Input: part model. Units: mm. Frame: model coordinates. Face numbers are marked on the shaded views. A direction names the side the tool comes from. Give positions to 0.01 mm unless a question says otherwise; leave off trailing zeros. Loops run counter-clockwise (first coordinate to the right, second up) from the corner with the lowest first, then second, coordinate; pieces in that order, holes last. Notation, with made-up numbers: (55, 26) -> (99, 26) arc R27 ccw to (99, 42) -> close; hole circle Ø8 at (35.25, 37.5). An arc over 180 degrees is marked (long way). Answer in a Markdown table with one row per item. Add a question column.
```python
from build123d import *

# Parameters (mm, degrees)
SKETCH1_R           = 2.25
BOSS_EXTRUDE1_DEPTH = 20
SKETCH2_R           = 2.25
BOSS_EXTRUDE2_DEPTH = 10
SKETCH4_W           = 26.5
SKETCH4_H           = 2.5
CUT_EXTRUDE1_DEPTH  = 39.17921555
CHAMFER2_SIZE       = 4
CHAMFER3_SIZE       = 4
FILLET4_R           = 2
SKETCH7_W           = 10
SKETCH7_H           = 10
BOSS_EXTRUDE5_DEPTH = 20
FILLET6_R           = 2
SKETCH8_W           = 63
SKETCH8_H           = 30
BOSS_EXTRUDE6_DEPTH = 4
CHAMFER4_SIZE       = 2
FILLET7_R           = 2


with BuildPart() as part:
    # Sketch1 → Boss-Extrude1 (new body)
    with BuildSketch(Plane(origin=(0, 0, 0), x_dir=(0, 0, -1), z_dir=(1, 0, 0))):
        Polygon((10.25, -20.3), (13.25, -20.3), (13.25, 29.7), (-13.25, 29.7), (-13.25, -20.3), (-10.25, -20.3), (-10.25, 20.3), (10.25, 20.3), align=None)
        with Locations((5, 24)):
            Circle(SKETCH1_R, mode=Mode.SUBTRACT)
        with Locations((-5, 24)):
            Circle(SKETCH1_R, mode=Mode.SUBTRACT)
    extrude(amount=BOSS_EXTRUDE1_DEPTH)

    # Sketch2 → Boss-Extrude2 (add)
    with BuildSketch(Plane.ZY):
        with Locations((-5, 24)):
            Circle(SKETCH2_R)
        with Locations((5, 24)):
            Circle(SKETCH2_R)
    extrude(amount=-BOSS_EXTRUDE2_DEPTH)

    # Sketch4 → Cut-Extrude1 (cut, through all)
    with BuildSketch(Plane(origin=(20, 0, 0), x_dir=(0, 0, -1), z_dir=(1, 0, 0))):
        with Locations((0, 28.45)):
            Rectangle(SKETCH4_W, SKETCH4_H)
    extrude(amount=-CUT_EXTRUDE1_DEPTH, mode=Mode.SUBTRACT)

    # Chamfer2
    chamfer2_edges = [part.edges().sort_by_distance(p)[0] for p in [
        (10, 27.2, -13.25),
    ]]
    chamfer(chamfer2_edges, length=CHAMFER2_SIZE)

    # Chamfer3
    chamfer3_edges = [part.edges().sort_by_distance(p)[0] for p in [
        (10, 27.2, 13.25),
    ]]
    chamfer(chamfer3_edges, length=CHAMFER3_SIZE)

    # Fillet4
    fillet4_edges = [part.edges().sort_by_distance(p)[0] for p in [
        (10, 27.2, -9.25),
        (10, 27.2, 9.25),
    ]]
    fillet(fillet4_edges, radius=FILLET4_R)

    # Sketch7 → Boss-Extrude5 (add)
    with BuildSketch(Plane(origin=(20, 0, 0), x_dir=(0, 0, -1), z_dir=(1, 0, 0))):
        with Locations((18.25, 6.423218073)):
            Rectangle(SKETCH7_W, SKETCH7_H)
    extrude(amount=-BOSS_EXTRUDE5_DEPTH)

    # Fillet6
    fillet6_edges = [part.edges().sort_by_distance(p)[0] for p in [
        (10, 1.423218073, -13.25),
        (10, 11.423218073, -13.25),
    ]]
    fillet(fillet6_edges, radius=FILLET6_R)

    # Sketch8 → Boss-Extrude6 (add)
    with BuildSketch(Plane(origin=(0, 0, -23.25), x_dir=(-1, 0, 0), z_dir=(0, 0, -1))):
        with Locations((-13.9, 6.423218073)):
            Rectangle(SKETCH8_W, SKETCH8_H)
    extrude(amount=BOSS_EXTRUDE6_DEPTH)

    # Chamfer4
    chamfer4_edges = [part.edges().sort_by_distance(p)[0] for p in [
        (45.4, 6.423218073, -23.25),
        (13.9, -8.576781927, -23.25),
        (-17.6, 6.423218073, -23.25),
        (13.9, 21.423218073, -23.25),
    ]]
    chamfer(chamfer4_edges, length=CHAMFER4_SIZE)

    # Fillet7
    fillet7_edges = [part.edges().sort_by_distance(p)[0] for p in [
        (10, 11.423218073, -23.25),
        (10, 1.423218073, -23.25),
    ]]
    fillet(fillet7_edges, radius=FILLET7_R)


solid = part.part
```
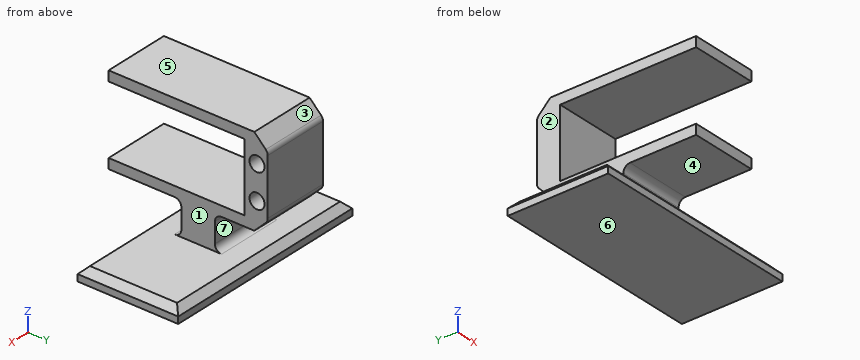
1) Pin query (flat end, axial travel): pin 1 (10 mm diameter, centred on x = 11.5, z = 0, fed in from -Y); pin 2 (1.3 mm diameter, centred on y = 23.5, z = -5, fed in from +X); pin 3 (11 mm diameter, centred on y = 2.5, z = -14, fed in from +X); pin 4 (2 mm diameter, centred on y = 19, z = -4.5, fed in from -X). Return the tip coordinate at first contact, or that it passes through.
2) Section B-B on z = -5. Output: boundary loops of the cut face in (x, y), and give its area (3 significant figures).
3) Pull-direction query (Z, two-part tool) for the marked faces 5, 6 and 7; classes: +Z half, -Z half, draft (parallel to the pull), parting line (faces both ways), or undercut.
4) Section A-A on y = 15. Output: boundary loops of the cut face in (x, z), and give its area (3 significant figures).
5) Section C-C on y = 24. Output: boundary loops of the cut face in (x, z), and give its area (3 significant figures).
6) Material intervals for line 1 along Y through (x, z) = (13.75, 5); line 2 along Z through (x, y) = (8.5, -15); line 3 along Z through (x, y) = (15.5, 24), sorted ascending.
7) Reachability of the marked faces 1, 2, 3 and 4 from +Z, -Z, +X, -X, +Y, -Y: full face, straight path, thin tool, end or side. Return the list, or none.
8) Section D-D on x = -12. Output: boundary loops of the cut face in (y, z), and give its area (3 significant figures).
Working result:
| question | item | result |
|---|---|---|
| 1 | pin 1 | stops at y = 20.3 |
| 1 | pin 2 | stops at x = 10 |
| 1 | pin 3 | stops at x = 20 |
| 1 | pin 4 | passes through |
| 2 | outline | (0, 20.3) -> (20, 20.3) -> (20, 21.75) -> (10, 21.75) -> (10, 26.25) -> (20, 26.25) -> (20, 27.2) -> (0, 27.2) -> close |
| 2 | area | 93.0 mm2 |
| 3 | face 5 | +Z half |
| 3 | face 6 | -Z half |
| 3 | face 7 | undercut |
| 4 | outline | (-17.6, -27.25) -> (45.4, -27.25) -> (45.4, -25.25) -> (43.4, -23.25) -> (-15.6, -23.25) -> (-17.6, -25.25) -> close; (0, -13.25) -> (20, -13.25) -> (20, -10.25) -> (0, -10.25) -> close; (0, 10.25) -> (20, 10.25) -> (20, 13.25) -> (0, 13.25) -> close |
| 4 | area | 368 mm2 |
| 5 | outline | (0, -12.45) -> (20, -12.45) -> (20, -7.25) -> (10, -7.25) -> (10, -2.75) -> (20, -2.75) -> (20, 2.75) -> (10, 2.75) -> (10, 7.25) -> (20, 7.25) -> (20, 12.45) -> (0, 12.45) -> close |
| 5 | area | 408 mm2 |
| 6 | line 1 | y = 20.3 to 21.75, 26.25 to 27.2 |
| 6 | line 2 | z = -13.25 to -10.25, 10.25 to 13.25 |
| 6 | line 3 | z = -12.45 to -7.25, -2.75 to 2.75, 7.25 to 12.45 |
| 7 | face 1 | +Z, +X, +Y, -Y |
| 7 | face 2 | +Z, -X, +Y, -Y |
| 7 | face 3 | +Z, +X, -X, +Y |
| 7 | face 4 | +X, -X, -Y |
| 8 | outline | (-8.58, -27.25) -> (21.42, -27.25) -> (21.42, -25.25) -> (19.42, -23.25) -> (-6.58, -23.25) -> (-8.58, -25.25) -> close |
| 8 | area | 116 mm2 |
